from build123d import *

# Parameters (mm, degrees)
SKETCH1_W           = 9.525
SKETCH1_H           = 3.175
BOSS_EXTRUDE1_DEPTH = 3.175
FILLET1_R           = 1


with BuildPart() as part:
    # Sketch1 → Boss-Extrude1 (new body)
    with BuildSketch(Plane.XY):
        with Locations((0, -8.6775)):
            Rectangle(SKETCH1_W, SKETCH1_H)
        Polygon((4.7625, 7.09), (-4.7625, 7.09), (-6.35, 7.09), (-6.35, -7.09), (-4.7625, -7.09), (4.7625, -7.09), (6.35, -7.09), (6.35, 7.09), align=None)
        with Locations((0, 8.6775)):
            Rectangle(SKETCH1_W, SKETCH1_H)
    extrude(amount=BOSS_EXTRUDE1_DEPTH)

    # Fillet1
    fillet1_edges = [part.edges().sort_by_distance(p)[0] for p in [
        (-6.35, -7.09, 1.5875),
        (-6.35, 7.09, 1.5875),
        (-4.7625, 10.265, 1.5875),
        (4.7625, 10.265, 1.5875),
        (6.35, 7.09, 1.5875),
        (6.35, -7.09, 1.5875),
        (4.7625, -10.265, 1.5875),
        (-4.7625, -10.265, 1.5875),
    ]]
    fillet(fillet1_edges, radius=FILLET1_R)


solid = part.part
Model file for the job. Use its own axes, mm. A direction names the side the tool comes from. Give positions to 0.01 mm unless a question says otherwise; leave off trailing zeros. Order: outer loops, then holes, each group sorted by start corner. A loop starts at its lowest first (then second) coordinate and runs counter-clockwise, first axis right, second up. Notation, with made-up numbers: (73.5, -29.75) - (87.5, -29.75) arc R7 ccw to (87.5, -22.75) - close; hole circle Ø2 at (4.5, 3.25). An arc over 180 degrees is marked (long way). One line per item, written item: value.
Item 1: Pin check, flat tips, straight feed: pin 1 Ø1.7 at (y, z) = (-8.5, 1.5) entering from -X; pin 2 Ø1.1 at (y, z) = (8.5, 1.5) entering from +X. Stop position of each tip, or through.
Response values:
pin 1: x = -4.76
pin 2: x = 4.76
Item 2: Slice it at B-B (y = -7.75). List the corners of the cut face in (x, z) (1 decimal).
Response values:
outline: (-4.8, 0) - (4.8, 0) - (4.8, 3.2) - (-4.8, 3.2) - close
Item 3: Tool access for faces 1 (the flat face through (-4.762, -8, 2)), 2 (the flat face through (4.762, 8, 2)), 3 (the flat face through (-4.762, 8, 2)): list every direction of +Z, -Z, +X, -X, +Y, -Y with a clear straight run to the whole face (end or side of a thin tool).
Response values:
face 1: +Z, -Z, -X, -Y
face 2: +Z, -Z, +X, +Y
face 3: +Z, -Z, -X, +Y
Item 4: Wall check: line 1 (X direction, y = 7.5, z = 0.8); line 2 (Y direction, x = -5, z = 1.05); line 3 (Y direction, x = 4.5, z = 2.9). Give the ranges that are in metal, low to high.
Response values:
line 1: -4.76 to 4.76
line 2: -7.09 to 7.09
line 3: -9.94 to 9.94
